Autodesk Inventor part; units mm, degrees
ref_plane "Work Plane1" through (0, 0, 44.45) normal (0, 0, 1) x (1, 0, 0)
ref_plane "Work Plane2" through (44.45, 0, 0) normal (1, 0, 0) x (0, 1, 0)
ref_plane "XZ Plane" through (0, 0, 0) normal (0, 1, 0) x (-1, 0, 0)
sketch "Sketch1" plane through (0, 0, 0) normal (0, 1, 0) x (-1, 0, 0)
  circle A0 centre (0, 0) radius 38.1
  circle A1 centre (0, 0) radius 44.45
  dimension "d0" = 76.2
  dimension "d1" = 88.9
extrude "Extrusion1" add sketch "Sketch1" along normal mid plane 25.4
ref_plane "Work Plane1" through (0, 0, 44.45) normal (0, 0, 1) x (1, 0, 0)
sketch "Sketch2" plane through (0, 0, 44.45) normal (0, 0, 1) x (1, 0, 0)
  point P0 (0, 0)
  point P1 (0, 0)
hole "Hole1" at (0, 0, 44.45) direction (0, 0, -1) diameter 6.35 end through all
ref_plane "Work Plane2" through (44.45, 0, 0) normal (1, 0, 0) x (0, 1, 0)
sketch "Sketch3" plane through (44.45, 0, 0) normal (1, 0, 0) x (0, 1, 0)
  point P0 (0, 0)
  point P1 (0, 0)
hole "Hole2" at (44.45, 0, 0) direction (-1, 0, 0) diameter 6.7564 end through all
equation "\"d0\" = cupDiam"
equation "\"d1\" = outerRingDism"
equation "\"d2\" = ringHeight"
equation "\"d5\" = ringAxelDiam"
equation "\"cupDiam\" = 76.2"
equation "\"ringThickness\" = 6.35"
equation "\"ringHeight\" = 25.4"
equation "\"ringAxelDiam\" = 6.35"
equation "\"outerRingDism\" = cupDiam + 2 * ringThickness"
equation "\"outerRingRadius\" = 0.5 * outerRingDism"
equation "\"d4\" = outerRingRadius"
equation "\"d12\" = outerRingRadius"
properties part number "RounedInnerRing"
The listing builds one solid part. Answer for the finished solid, in the listing's coordinates (mm). Coordinates: 2 decimals unless noted, no trailing zeros. Write each loop counter-clockwise with the first axis right and the second up, starting at its lowest first coordinate (ties: lowest second). Pieces come first, ordered by that corner, then holes. Notation, with made-up numbers: (37, -2.75) - (53, -2.75) arc R22 cw to (53, 24.25) - close; hole circle Ø9 at (65.25, -19.5). An arc over 180 degrees is marked (long way). Return JSON: item names as keys, results as strings.
1. Each of these flat-tipped pins is pushed along its axis until it touches: pin 1 Ø1 at (y, z) = (-3.5, -9) entering from -X; pin 2 Ø4 at (x, y) = (18.5, -7) entering from +Z; pin 3 Ø12 at (y, z) = (9, -14.5) entering from +X. Where does it stop, or does it pass through?
Final values:
{"pin 1": "x = -43.63", "pin 2": "z = 41.27", "pin 3": "x = 43.63"}
2. Consider line 1 along Y through (x, z) = (0, 42.5) (3 decimals); line 2 along X through (y, z) = (0.5, 23.5); line 3 along X through (y, z) = (-3.75, 5.5). Determine where each line is inside the solid, lowest interval first.
Final values:
{"line 1": "-12.7 to -3.175, 3.175 to 12.7", "line 2": "-37.73 to -29.99, 29.99 to 37.73", "line 3": "-44.11 to -37.7, 37.7 to 44.11"}
3. The part is cut by section C-C on x = 12. Determine the outline of the cut face in (y, z), then the cut area to 3 significant figures.
Final values:
{"outline": "(-12.7, -42.8) - (12.7, -42.8) - (12.7, -36.16) - (-12.7, -36.16) - close; (-12.7, 36.16) - (12.7, 36.16) - (12.7, 42.8) - (-12.7, 42.8) - close", "area": "337 mm^2"}
4. For a pull along Y with two mould halves and no side action, classify faces 1 (the face through (3.1, 0.69, 41.16)), 2 (the face through (-33, -12.7, 20)), 3 (the face through (-33, 12.7, 20)) as +Y half, -Y half, draft (parallel to the pull), parting line (faces both ways), or undercut.
Final values:
{"face 1": "undercut", "face 2": "-Y half", "face 3": "+Y half"}
5. The part is cut by section D-D on z = 27. Determine the outline of the cut face in (x, y).
Final values:
{"outline": "(-35.31, -12.7) - (-26.88, -12.7) - (-26.88, 12.7) - (-35.31, 12.7) - close; (26.88, -12.7) - (35.31, -12.7) - (35.31, 12.7) - (26.88, 12.7) - close"}
6. The part is cut by section A-A on x = 0. Determine the outline of the cut face in (y, z) (3 decimals), then the cut area to 3 significant figures.
Final values:
{"outline": "(-12.7, -44.45) - (-3.175, -44.45) - (-3.175, -38.1) - (-12.7, -38.1) - close; (-12.7, 38.1) - (-3.175, 38.1) - (-3.175, 44.45) - (-12.7, 44.45) - close; (3.175, -44.45) - (12.7, -44.45) - (12.7, -38.1) - (3.175, -38.1) - close; (3.175, 38.1) - (12.7, 38.1) - (12.7, 44.45) - (3.175, 44.45) - close", "area": "242 mm^2"}
7. The part is cut by section B-B on z = 0. Determine the outline of the cut face in (x, y).
Final values:
{"outline": "(-44.45, -12.7) - (-38.1, -12.7) - (-38.1, -3.38) - (-44.45, -3.38) - close; (-44.45, 3.38) - (-38.1, 3.38) - (-38.1, 12.7) - (-44.45, 12.7) - close; (38.1, -12.7) - (44.45, -12.7) - (44.45, -3.38) - (38.1, -3.38) - close; (38.1, 3.38) - (44.45, 3.38) - (44.45, 12.7) - (38.1, 12.7) - close"}
